```python
from build123d import *

# Parameters (mm, degrees)
BRACKET_DEPTH = 11.5


with BuildPart() as part:
    # Sketch9 → Bracket (new body)
    with BuildSketch(Plane(origin=(0, 0, 0), x_dir=(1, 0, 0), z_dir=(0, 1, 0))):
        with BuildLine():
            Line((5.15, -5), (4.65, -5))
            Line((4.65, -5), (3.35, -5))
            Line((3.35, -5), (3.35, -7))
            Line((3.35, -7), (6.4, -7))
            ThreePointArc((6.4, -7), (6.930330086, -6.780330086), (7.15, -6.25))
            Line((7.15, -6.25), (7.15, -5))
            Line((7.15, -5), (7.15, -3.25))
            ThreePointArc((7.15, -3.25), (7.369669914, -2.719669914), (7.9, -2.5))
            Line((7.9, -2.5), (21.4, -2.5))
            ThreePointArc((21.4, -2.5), (21.930330086, -2.280330086), (22.15, -1.75))
            Line((22.15, -1.75), (22.15, 24.75))
            ThreePointArc((22.15, 24.75), (21.930330086, 25.280330086), (21.4, 25.5))
            Line((21.4, 25.5), (7.9, 25.5))
            ThreePointArc((7.9, 25.5), (7.369669914, 25.719669914), (7.15, 26.25))
            Line((7.15, 26.25), (7.15, 28))
            Line((7.15, 28), (7.15, 29.75))
            ThreePointArc((7.15, 29.75), (6.930330086, 30.280330086), (6.4, 30.5))
            Line((6.4, 30.5), (5.15, 30.5))
            Line((5.15, 30.5), (3.35, 30.5))
            Line((3.35, 30.5), (3.35, 28.5))
            Line((3.35, 28.5), (5.15, 28.5))
            Line((5.15, 28.5), (5.15, 28))
            Line((5.15, 28), (5.15, 23.5))
            Line((5.15, 23.5), (20.15, 23.5))
            Line((20.15, 23.5), (20.15, -0.5))
            Line((20.15, -0.5), (5.15, -0.5))
            Line((5.15, -0.5), (5.15, -5))
        make_face()
    extrude(amount=BRACKET_DEPTH)


solid = part.part
```
Here's how the part is built. I have some questions about the finished solid (model axes, mm). A direction names the side the tool comes from. Coordinates: 2 decimals unless noted, no trailing zeros. Order: outer loops, then holes, each group sorted by start corner. A loop starts at its lowest first (then second) coordinate and runs counter-clockwise, first axis right, second up. Notation, with made-up numbers: M -34,54 L -27,54 A23 ccw -27,92 Z; hole C 48,-27 d1. An arc over 180 degrees is marked long. Answer as a JSON object with one key per item and string values. Group by question number.
(1) I need wall thicknesses on probe 1 along Z at (x, y) = (9.75, 3.75); probe 2 along Z at (x, y) = (5, 9.5); probe 3 along X at (y, z) = (7.25, -19). Which ranges of each line are inside material? Lowest first, please.
(2) Suppose I cut it at C-C, the plane x = 6.75. Please give me the cut outline in (y, z), then the cut area to 3 significant figures.
(3) Which directions (+Z, -Z, +X, -X, +Y, -Y) give clear straight access to the entire face, cutting with the end or side of a thin tool? Please do faces 5 (the face through (3.35, 6, 6)), 6 (the face through (15, 6, -25.5)), 7 (the face through (13, 6, 0.5)), 8 (the face through (7.15, 6, 5)).
(4) Suppose I cut it at D-D, the plane z = -1.5. Please give me the cut outline in (x, y), then the cut area to 3 significant figures.
(5) Suppose I cut it at B-B, the plane y = 9.5. Please give me the cut outline in (x, z).
(6) Suppose I cut it at A-A, the plane x = 16. Please give me the cut outline in (y, z), then the cut area to 3 significant figures.
(7) If we mould it in two halves opening along Z, with no side actions, what happens to faces 1 (the face through (5, 6, -30.5)), 2 (the face through (13, 6, -23.5)), 3 (the face through (15, 6, 2.5)), 4 (the face through (20.4, 0, -10.4))? For each: released by +Z, released by -Z, zero draft, split by the parting line, or undercut.
(8) For pin 1 (4 mm diameter, centred on y = 10, z = -18.5, fed in from -X); pin 2 (2.5 mm diameter, centred on y = 6, z = 5, fed in from +X); pin 3 (2.5 mm diameter, centred on y = 8.5, z = -25, fed in from -X), each with a flat end and sliding along its axis, tell me the tip position at first contact or that it passes through.
Values found:
{
 "1": {"probe 1": "z = -25.5 to -23.5, 0.5 to 2.5", "probe 2": "z = -30.5 to -28.5, 5 to 7", "probe 3": "x = 20.15 to 22.15"},
 "2": {"outline": "M 0,-30.41 L 11.5,-30.41 L 11.5,-23.5 L 0,-23.5 Z; M 0,0.5 L 11.5,0.5 L 11.5,6.91 L 0,6.91 Z", "area": "153 mm^2"},
 "3": {"face 5": "+Z, -Z, -X, +Y, -Y", "face 6": "-Z, +X, +Y, -Y", "face 7": "-X, +Y, -Y", "face 8": "+Z, +X, +Y, -Y"},
 "4": {"outline": "M 20.15,0 L 22.15,0 L 22.15,11.5 L 20.15,11.5 Z", "area": "23.0 mm^2"},
 "5": {"outline": "M 3.35,-30.5 L 6.4,-30.5 A0.75 ccw 7.15,-29.75 L 7.15,-26.25 A0.75 cw 7.9,-25.5 L 21.4,-25.5 A0.75 ccw 22.15,-24.75 L 22.15,1.75 A0.75 ccw 21.4,2.5 L 7.9,2.5 A0.75 cw 7.15,3.25 L 7.15,6.25 A0.75 ccw 6.4,7 L 3.35,7 L 3.35,5 L 5.15,5 L 5.15,0.5 L 20.15,0.5 L 20.15,-23.5 L 5.15,-23.5 L 5.15,-28.5 L 3.35,-28.5 Z"},
 "6": {"outline": "M 0,-25.5 L 11.5,-25.5 L 11.5,-23.5 L 0,-23.5 Z; M 0,0.5 L 11.5,0.5 L 11.5,2.5 L 0,2.5 Z", "area": "46.0 mm^2"},
 "7": {"face 1": "released by -Z", "face 2": "undercut", "face 3": "released by +Z", "face 4": "zero draft"},
 "8": {"pin 1": "stops at x = 20.15", "pin 2": "stops at x = 7.15", "pin 3": "stops at x = 5.15"}
}
